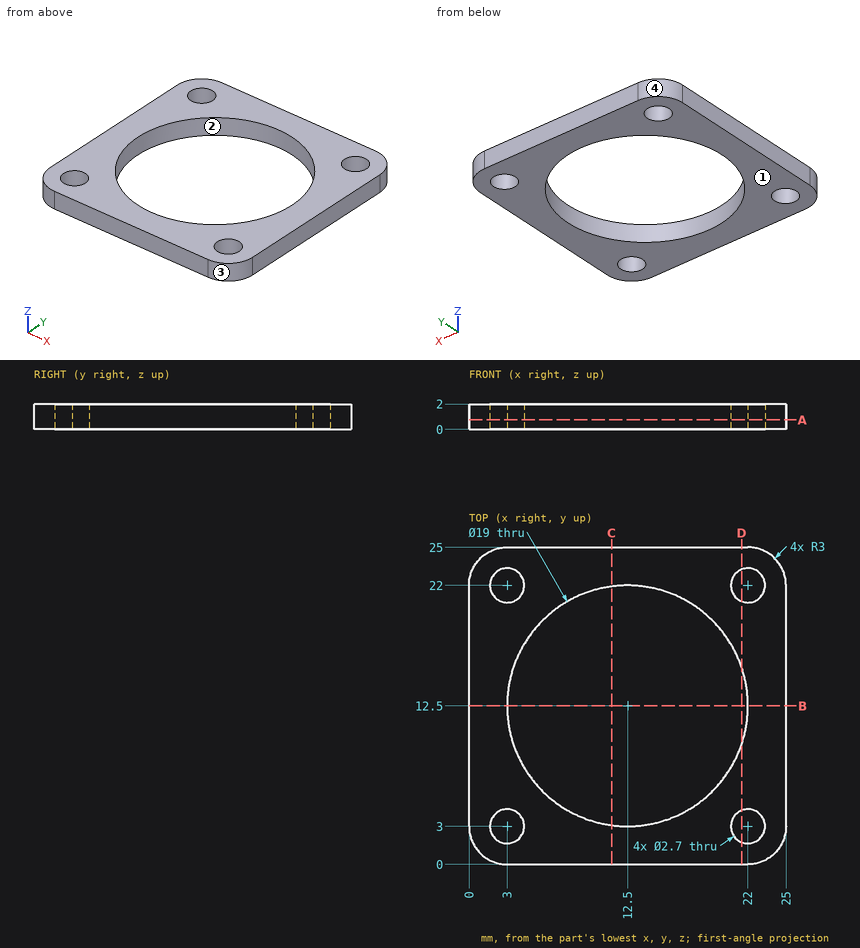
Here's the drawing with two shaded views (mm, measured from the low corner). I have some questions. Coordinates: 2 decimals unless noted, no trailing zeros. Loops run counter-clockwise (first coordinate to the right, second up) from the corner with the lowest first, then second, coordinate; pieces in that order, holes last. Notation, with made-up numbers: M 88.25,-28 L 134.25,-28 A14 ccw 134.25,-8 Z; hole C -27.5,50 d9. An arc over 180 degrees is marked long. Return JSON: item names as keys, results as strings. Group by question number.
Item 1: Imagine slicing it at B-B (y = 12.5). Please give me the cut outline in (x, z).
Item 2: If I drill on L1, parallel to X at y = 2.25, z = 1.05; L2, parallel to Y at x = 12.5, z = 0.7; L3, parallel to Y at x = 21.25, z = 1.9, over which ranges is the centre line in solid material (lowest first)? Write a range as from..to.
Item 3: Thinking about a two-plate mould opening in X: for the marked faces 1, 2, 3 and 4, which applies, released by +X, released by -X, zero draft, split by the parting line, or undercut?
Item 4: Imagine slicing it at C-C (x = 11.25). Please give me the cut outline in (y, z).
Item 5: Imagine slicing it at D-D (x = 21.5). Please give me the cut outline in (y, z), and give its area (3 significant figures).
Item 6: Imagine slicing it at A-A (z = 0.75). Please give me the cut outline in (x, y), and give its area (3 significant figures).
Verdict:
{
 "1": {"outline": "M 0,0 L 3,0 L 3,2 L 0,2 Z; M 22,0 L 25,0 L 25,2 L 22,2 Z"},
 "2": {"L1": "x = 0.1..1.88, 4.12..20.88, 23.12..24.9", "L2": "y = 0..3, 22..25", "L3": "y = 0..1.88, 4.12..8.8, 16.2..20.88, 23.12..25"},
 "3": {"face 1": "zero draft", "face 2": "undercut", "face 3": "released by +X", "face 4": "released by -X"},
 "4": {"outline": "M 0,0 L 3.08,0 L 3.08,2 L 0,2 Z; M 21.92,0 L 25,0 L 25,2 L 21.92,2 Z"},
 "5": {"outline": "M 0,0 L 1.75,0 L 1.75,2 L 0,2 Z; M 4.25,0 L 9.46,0 L 9.46,2 L 4.25,2 Z; M 15.54,0 L 20.75,0 L 20.75,2 L 15.54,2 Z; M 23.25,0 L 25,0 L 25,2 L 23.25,2 Z", "area": "27.8 mm^2"},
 "6": {"outline": "M 0,3 A3 ccw 3,0 L 22,0 A3 ccw 25,3 L 25,22 A3 ccw 22,25 L 3,25 A3 ccw 0,22 Z; hole C 3,3 d2.7; hole C 3,22 d2.7; hole C 12.5,12.5 d19; hole C 22,3 d2.7; hole C 22,22 d2.7", "area": "311 mm^2"}
}
